Source: three-view drawing plus pictorial views. Frame: mm from the lowest corner of the part. Give positions to 0.01 mm unless a question says otherwise; leave off trailing zeros. Order: outer loops, then holes, each group sorted by start corner. A loop starts at its lowest first (then second) coordinate and runs counter-clockwise, first axis right, second up. Notation, with made-up numbers: (66, 72.5) -> (72, 72.5) arc R18 cw to (72, 94.5) -> close; hole circle Ø8 at (44.25, 43.5). An arc over 180 degrees is marked (long way). One line per question, with ' | ' between items.
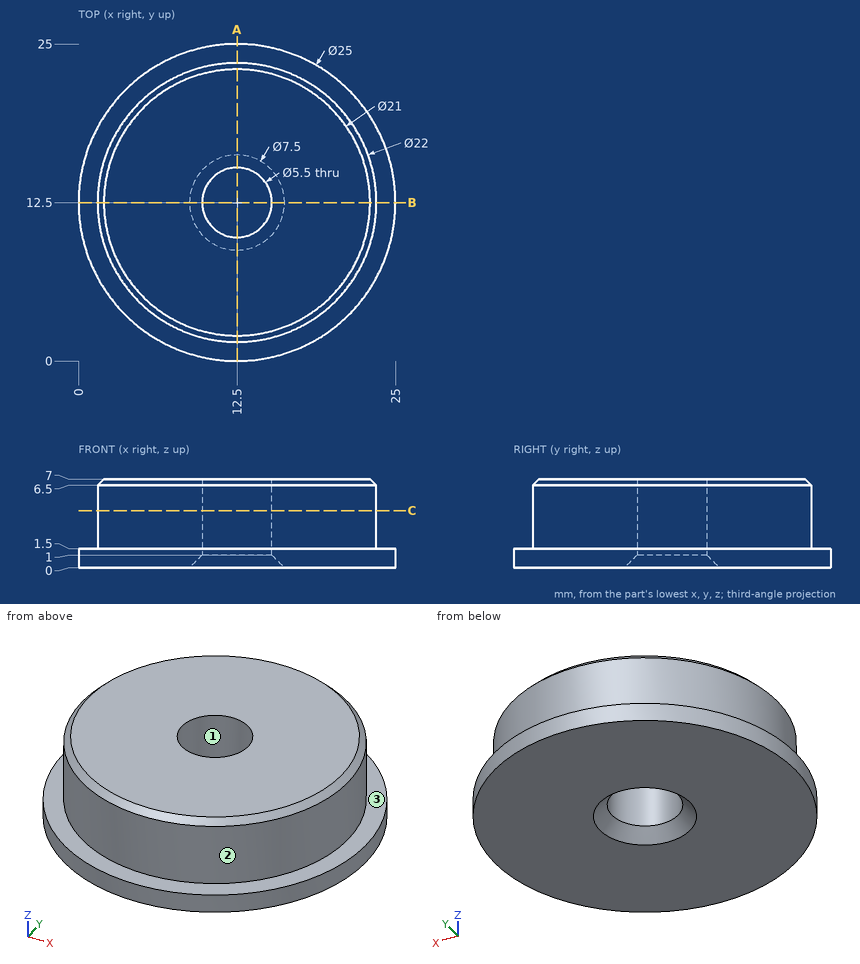
1) Pull-direction query (Y, two-part tool) for the marked faces 1, 2 and 3; classes: +Y half, -Y half, draft (parallel to the pull), parting line (faces both ways), or undercut.
Check result:
face 1: undercut | face 2: parting line | face 3: draft
2) Contact query for flat-ended pins moving along their axis: pin 1 Ø2 at (x, z) = (16, 1.5) entering from +Y; pin 2 Ø3 at (y, z) = (9, 4.5) entering from -X. Output: stop coordinate, or through.
Check result:
pin 1: stops at y = 24.75 | pin 2: stops at x = 1.68
3) Section C-C on z = 4.5. Return loops of the section in (x, y).
Check result:
outline: circle Ø22 at (12.5, 12.5); hole circle Ø5.5 at (12.5, 12.5)
4) Section A-A on x = 12.5. Return loops of the section in (y, z).
Check result:
outline: (0, 0) -> (8.75, 0) -> (9.75, 1) -> (9.75, 7) -> (2, 7) -> (1.5, 6.5) -> (1.5, 1.5) -> (0, 1.5) -> close; (15.25, 1) -> (16.25, 0) -> (25, 0) -> (25, 1.5) -> (23.5, 1.5) -> (23.5, 6.5) -> (23, 7) -> (15.25, 7) -> close
5) Material intervals for probe 1 along Y at (x, z) = (12.5, 4.5); probe 2 along Z at (x, y) = (22.5, 6); probe 3 along X at (y, z) = (12.75, 0.75), sorted ascending. Write a range as from..to.
Check result:
probe 1: y = 1.5..9.75, 15.25..23.5 | probe 2: z = 0..1.5 | probe 3: x = 0..9.51, 15.49..25
